Verification items for the finished model (mm, model axes). Give positions to 0.01 mm unless a question says otherwise; leave off trailing zeros. Order: outer loops, then holes, each group sorted by start corner. A loop starts at its lowest first (then second) coordinate and runs counter-clockwise, first axis right, second up.
(1) Gauge pin test, flat ends, axial feed: pin 1 (7 mm diameter, centred on x = 260, y = 10, fed in from -Z); pin 2 (4.5 mm diameter, centred on x = 260, y = 70, fed in from -Z). Record the tip position at first contact, or that the pin passes through.
(2) Scan lines: L1, parallel to Y at x = 260, z = 3; L2, parallel to X at y = 10, z = 3.7; L3, parallel to X at y = 11, z = 3.9. Record each from-to range of solid material in increasing order.
(3) Mould release check, pull along Y, two halves, no side actions. Record for faces 1 (the face through (137, 80, 2)), 2 (the face through (0, 41, 2)), 3 (the face through (9.879, 72.747, 2.465)): pulls with the +Y half, pulls with the -Y half, needs draft (parallel to the pull), parting line crosses it, or undercut.
(4) Sectioned sample at A-A on x = 10. Record the cut outline in (y, z).
(5) Sectioned sample at B-B on y = 10. Record the cut outline in (x, z), plus the area to 4 significant figures.
Autodesk Inventor part; units mm, degrees
ref_plane "YZ Plane" through (0, 0, 0) normal (1, 0, 0) x (0, 1, 0)
ref_plane "XZ Plane" through (0, 0, 0) normal (0, 1, 0) x (-1, 0, 0)
ref_plane "XY Plane" through (0, 0, 0) normal (0, 0, 1) x (1, 0, 0)
sketch "Sketch1" plane through (0, 0, 0) normal (0, 0, 1) x (1, 0, 0)
  line L0 (0, 0) -> (270, 0)
  line L1 (270, 0) -> (270, 80)
  line L2 (270, 80) -> (0, 80)
  line L3 (0, 80) -> (0, 0)
  dimension "d2" = 80
  dimension "d3" = 270
extrude "Extrusion1" add sketch "Sketch1" along normal blind 5
sketch "Sketch2" plane through (0, 0, 5) normal (0, 0, 1) x (1, 0, 0)
  circle A0 centre (10, 70) radius 2.75
  circle A1 centre (260, 70) radius 2.75
  circle A2 centre (260, 10) radius 2.75
  circle A3 centre (10, 10) radius 2.75
  line L0 (270, 80) -> (0, 80)
  line L1 (0, 80) -> (0, 0)
  line L2 (270, 0) -> (270, 80)
  line L3 (0, 0) -> (270, 0)
  dimension "d4" = 10
  dimension "d5" = 10
  dimension "d6" = 10
  dimension "d7" = 10
  dimension "d8" = 10
  dimension "d9" = 10
  dimension "d10" = 10
  dimension "d11" = 10
  dimension "d12" = 5.5
  dimension "d13" = 5.5
  dimension "d14" = 5.5
  dimension "d15" = 5.5
hole "Hole1" at (10, 70, 5) at (10, 10, 5) at (260, 10, 5) at (260, 70, 5) direction (0, 0, -1) diameter 5.5 end through all
fillet "Fillet1" radius 2 4 edges at (0, 80, 2.5) (270, 80, 2.5) (270, 0, 2.5) (0, 0, 2.5)
equation "\"d5\" = d4"
equation "\"d6\" = d4"
equation "\"d7\" = d4"
equation "\"d8\" = d4"
equation "\"d9\" = d4"
equation "\"d10\" = d4"
equation "\"d11\" = d4"
equation "\"d13\" = d12"
equation "\"d14\" = d12"
equation "\"d15\" = d12"
equation "\"d16\" = d12"
properties part number "HeightPlates"
Ans:
1. pin 1: stops at z = 0
1. pin 2: passes through
2. L1: y = 0 to 7.25, 12.75 to 67.25, 72.75 to 80
2. L2: x = 0 to 7.25, 12.75 to 257.25, 262.75 to 270
2. L3: x = 0 to 7.44, 12.56 to 257.44, 262.56 to 270
3. face 1: pulls with the +Y half
3. face 2: needs draft
3. face 3: undercut
4. outline: (0, 0) - (7.25, 0) - (7.25, 5) - (0, 5) - close; (12.75, 0) - (67.25, 0) - (67.25, 5) - (12.75, 5) - close; (72.75, 0) - (80, 0) - (80, 5) - (72.75, 5) - close
5. outline: (0, 0) - (7.25, 0) - (7.25, 5) - (0, 5) - close; (12.75, 0) - (257.25, 0) - (257.25, 5) - (12.75, 5) - close; (262.75, 0) - (270, 0) - (270, 5) - (262.75, 5) - close
5. area: 1,295 mm2
